Autodesk Inventor part; units mm, degrees
ref_plane "YZ Plane" through (0, 0, 0) normal (1, 0, 0) x (0, 1, 0)
ref_plane "XZ Plane" through (0, 0, 0) normal (0, 1, 0) x (-1, 0, 0)
ref_plane "XY Plane" through (0, 0, 0) normal (0, 0, 1) x (1, 0, 0)
ref_plane "工作平面1" through (0, 0, 0) normal (0, -1, 0) x (1, 0, 0)
sketch "草图2" plane through (0, 0, 0) normal (0, -1, 0) x (1, 0, 0)
  line L0 (13.9089, -43.2782) -> (-26.0911, -43.2782)
  arc A0 (13.9089, -43.2782) -> (21.4089, -35.7782) centre (13.9089, -35.7782) ccw
  line L1 (-33.5911, -35.7782) -> (21.4089, -35.7782)
  arc A1 (-33.5911, -35.7782) -> (-26.0911, -43.2782) centre (-26.0911, -35.7782) ccw
  point P0 (0, 0)
extrude "拉伸2" add sketch "草图2" along normal blind 2
ref_plane "工作平面2" through (-1.2405, 0, -40.1772) normal (0, -1, 0) x (1, 0, 0)
sketch "草图3" plane through (0, -2, 0) normal (0, -1, 0) x (1, 0, 0)
  line L0 (-21.0911, -35.7782) -> (8.9089, -35.7782)
  line L1 (8.9089, -35.7782) -> (8.9089, -43.7782)
  line L2 (8.9089, -43.7782) -> (-21.0911, -43.7782)
  line L3 (21.4089, -35.7782) -> (-33.5911, -35.7782)
  line L4 (-21.0911, -38.7782) -> (-19.5911, -38.7782)
  line L5 (-19.5911, -38.7782) -> (-19.5911, -39.7782)
  line L6 (-19.5911, -39.7782) -> (-21.0911, -39.7782)
  line L7 (-21.0911, -43.7782) -> (-21.0911, -39.7782)
  line L8 (-21.0911, -38.7782) -> (-21.0911, -35.7782)
  line L9 (8.9089, -39.7782) -> (7.4089, -39.7782)
  line L10 (7.4089, -39.7782) -> (7.4089, -38.7782)
  line L11 (7.4089, -38.7782) -> (8.9089, -38.7782)
  line L12 (8.9089, -38.7782) -> (8.9089, -39.7782)
  point P0 (0, 0)
  dimension "d7" = 8
  dimension "d8" = 1
  dimension "d9" = 3
  dimension "d10" = 1.5
  dimension "d11" = 1.5
extrude "拉伸3" add sketch "草图3" along normal blind 345 contours L0 L1 L11 L10 L9 L2 L7 L6 L5 L4 L8
ref_plane "工作平面3" through (0, -174.5, 0) normal (0, -1, 0) x (1, 0, 0)
mirror "镜像1" about plane through (0, -174.5, 0) normal (0, -1, 0) of "拉伸2"
properties part number "导轨"
For this review, take the finished solid that the model builds, in its own axes (mm). Round coordinates to 2 decimals unless told otherwise and drop trailing zeros. Order: outer loops, then holes, each group sorted by start corner. A loop starts at its lowest first (then second) coordinate and runs counter-clockwise, first axis right, second up. Notation, with made-up numbers: (0, -14) -> (14, -14) arc R7 cw to (14, -1) -> close; hole circle Ø5 at (-40, -35). An arc over 180 degrees is marked (long way). Use a Markdown table: item, result.
Item 1: Take a section at A-A (x = -29). State the section outline as (y, z) points, plus the area to 3 significant figures.
Resolved:
| item | result |
|---|---|
| outline | (-349, -42.69) -> (-347, -42.69) -> (-347, -35.78) -> (-349, -35.78) -> close; (-2, -42.69) -> (0, -42.69) -> (0, -35.78) -> (-2, -35.78) -> close |
| area | 27.7 mm² |
Item 2: Take a section at B-B (y = -262.5). State the section outline as (x, z) points.
Resolved:
| item | result |
|---|---|
| outline | (-21.09, -43.78) -> (8.91, -43.78) -> (8.91, -39.78) -> (7.41, -39.78) -> (7.41, -38.78) -> (8.91, -38.78) -> (8.91, -35.78) -> (-21.09, -35.78) -> (-21.09, -38.78) -> (-19.59, -38.78) -> (-19.59, -39.78) -> (-21.09, -39.78) -> close |
Item 3: For line 1 along Y through (x, z) = (19, -40.75); line 2 along X through (y, z) = (-290.5, -42); line 3 along X through (y, z) = (-111.5, -39), list the stretches that pass through material, from the lowest coordinate up. Write a range as [from, to].
Resolved:
| item | result |
|---|---|
| line 1 | y = [-349, -347], [-2, 0] |
| line 2 | x = [-21.09, 8.91] |
| line 3 | x = [-19.59, 7.41] |
Item 4: Draft analysis for pull direction Y (two halves, no side actions). For faces 1 (the flat face through (-6, -349, -39)), 2 (the flat face through (14, -2, -39)), 3 (the flat face through (-6, 0, -39)), 4 (the cylindrical face through (-31.452, -348.014, -41.023)), state which applies: +Y half, -Y half, draft (parallel to the pull), parting line (faces both ways), or undercut.
Resolved:
| item | result |
|---|---|
| face 1 | -Y half |
| face 2 | undercut |
| face 3 | +Y half |
| face 4 | draft |
Item 5: Take a section at C-C (z = -41). State the section outline as (x, y) points, plus the area to 3 significant figures.
Resolved:
| item | result |
|---|---|
| outline | (-31.47, -349) -> (19.29, -349) -> (19.29, -347) -> (8.91, -347) -> (8.91, -2) -> (19.29, -2) -> (19.29, 0) -> (-31.47, 0) -> (-31.47, -2) -> (-21.09, -2) -> (-21.09, -347) -> (-31.47, -347) -> close |
| area | 10,600 mm² |
Item 6: For pin 1 (1.2 mm diameter, centred on y = -200.5, z = -42.5, fed in from +X); pin 2 (2.5 mm diameter, centred on y = -200.5, z = -37.5, fed in from -X); pin 3 (0.6 mm diameter, centred on x = -1, y = -348.5, fed in from -Z), all flat-tipped, find the tip position at first contact; note any pin that passes through.
Resolved:
| item | result |
|---|---|
| pin 1 | stops at x = 8.91 |
| pin 2 | stops at x = -21.09 |
| pin 3 | stops at z = -43.28 |
